Input: dimensioned drawing with shaded views. Units: mm. Origin: part minimum x, y, z. Round coordinates to 2 decimals unless told otherwise and drop trailing zeros. Order: outer loops, then holes, each group sorted by start corner. A loop starts at its lowest first (then second) coordinate and runs counter-clockwise, first axis right, second up. Notation, with made-up numbers: M -32.75,80 L 11.25,80 A16 cw 11.25,95 Z; hole C 81.25,41.25 d10. An arc over 180 degrees is marked long. Use one line per item in the form item = value. Start each with the question number.
Q1. Section B-B (x = 18.25). Return the cut outline in (y, z) (1 decimal).
Q2. Section C-C (z = 0.5). Give the number of separate pieces and of enclosed holes in the cut face, plus the area to 3 significant figures.
Q3. Pull-direction query (X, two-part tool) for the marked faces 1, 2 and 3; classes: pulls with the +X half, pulls with the -X half, needs draft (parallel to the pull), parting line crosses it, or undercut.
Q4. Contact query for a flat-ended pin moving along its axis: pin 1 (2 mm diameter, centred on x = 8, y = 5.5, fed in from +Z). Output: stop coordinate, or through.
Q5. Section A-A (y = 3.5). Return the cut outline in (x, z) (1 decimal).
Q6. Material intervals for probe 1 along X at (y, z) = (4, 2.55); probe 2 along Y at (x, z) = (20, 0.9) (1 decimal); probe 3 along Y at (x, z) = (20.5, 0.35) (1 decimal), sorted ascending.
Q7. Section D-D (y = 6.5). Return the cut outline in (x, z) (1 decimal).
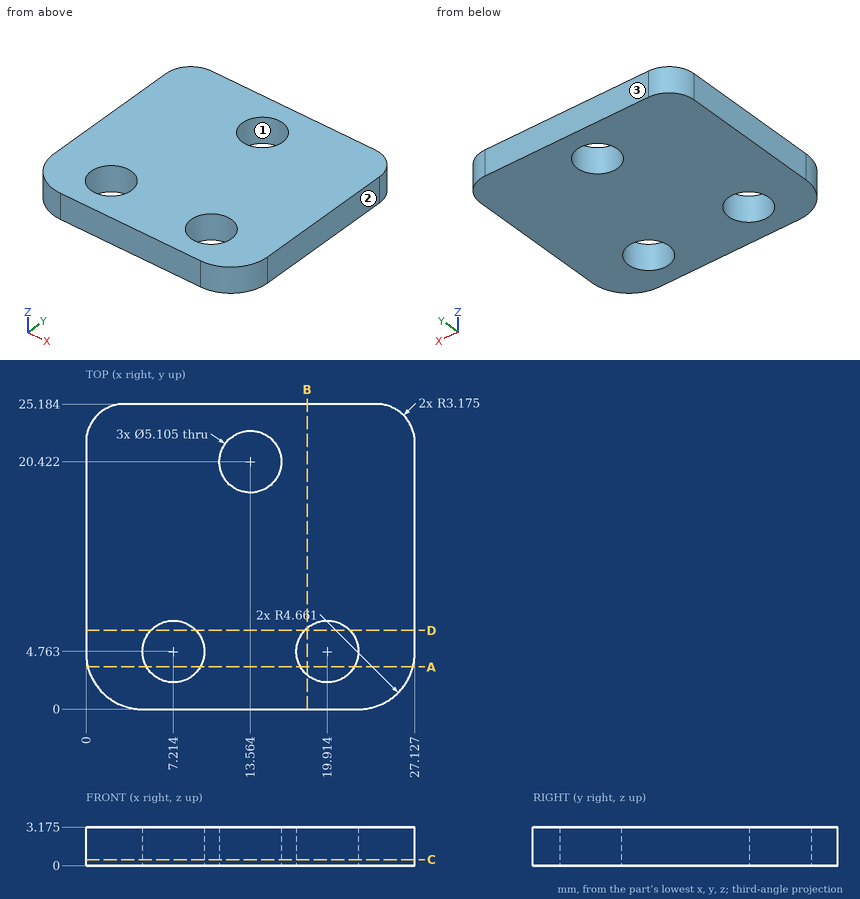
Results list:
q1.outline = M 0,0 L 2.8,0 L 2.8,3.2 L 0,3.2 Z; M 6.7,0 L 25.2,0 L 25.2,3.2 L 6.7,3.2 Z
q2.separate_pieces = 1
q2.enclosed_holes = 3
q2.area = 608 mm2
q3.face_1 = undercut
q3.face_2 = pulls with the +X half
q3.face_3 = needs draft
q4.pin_1 = through
q5.outline = M 0.1,0 L 5,0 L 5,3.2 L 0.1,3.2 Z; M 9.4,0 L 17.7,0 L 17.7,3.2 L 9.4,3.2 Z; M 22.1,0 L 27,0 L 27,3.2 L 22.1,3.2 Z
q6.probe_1 = 0.05 to 4.78, 9.65 to 17.48, 22.35 to 27.08
q6.probe_2 = 0 to 2.2, 7.3 to 25.2
q6.probe_3 = 0 to 2.3, 7.2 to 25.2
q7.outline = M 0,0 L 5.3,0 L 5.3,3.2 L 0,3.2 Z; M 9.1,0 L 18,0 L 18,3.2 L 9.1,3.2 Z; M 21.8,0 L 27.1,0 L 27.1,3.2 L 21.8,3.2 Z
